```python
from build123d import *

# Parameters (mm, degrees)
F1_DEPTH = 10
F2_R     = 4
F3_R     = 2
F4_DEPTH = 13


with BuildPart() as f1:
    # F0 (on Top) → F1 (new body)
    with BuildSketch(Plane.XY):
        with BuildLine():
            Line((44.1, 0), (71.5, 0))
            ThreePointArc((71.5, 0), (0, 30), (-71.5, 0))
            Line((-71.5, 0), (-44.1, 0))
            Line((-44.1, 0), (-44.1, 8.484979))
            ThreePointArc((-44.1, 8.484979), (0, 20), (44.1, 8.484979))
            Line((44.1, 8.484979), (44.1, 0))
        make_face()
    extrude(amount=F1_DEPTH)

    # F2
    f2_edges = [f1.edges().sort_by_distance(p)[0] for p in [
        (0, 20, 10),
        (0, 30, 10),
        (0, 20, 0),
        (0, 30, 0),
        (-44.1, 4.24249, 0),
        (-44.1, 4.24249, 10),
        (44.1, 4.24249, 0),
        (44.1, 4.24249, 10),
    ]]
    fillet(f2_edges, radius=F2_R)

    # F3 (on face) → F4 (cut)
    with BuildSketch(Plane.XZ):
        with Locations((48, 5)):
            Circle(F3_R)
        with Locations((-48, 5)):
            Circle(F3_R)
    extrude(amount=-F4_DEPTH, mode=Mode.SUBTRACT)


solid = f1.part
```
Verification items for the finished model (mm, model axes). A direction names the side the tool comes from. Coordinates: 2 decimals unless noted, no trailing zeros. Order: outer loops, then holes, each group sorted by start corner. A loop starts at its lowest first (then second) coordinate and runs counter-clockwise, first axis right, second up. Notation, with made-up numbers: (-32.5, 27) - (21.5, 27) arc R29 ccw to (21.5, 51) - close; hole circle Ø5 at (40, 56.5). An arc over 180 degrees is marked (long way). Return JSON: item names as keys, results as strings.
(1) Section check A-A, the plane y = 6. Give the number of separate pieces and of enclosed holes in the cut face, and give its area (3 significant figures).
Filled sheet:
{"separate pieces": "2", "enclosed holes": "2", "area": "359 mm^2"}
(2) Thickness scan on line 1 along Z through (x, y) = (-48, 6); line 2 along X through (y, z) = (8, 6.75); line 3 along X through (y, z) = (3, 9). Record the ranges inside material, lowest first.
Filled sheet:
{"line 1": "z = 0 to 3, 7 to 10", "line 2": "x = -62.54 to -48.97, -47.03 to -44.17, 44.17 to 47.03, 48.97 to 62.54", "line 3": "x = -66.43 to -45.45, 45.45 to 66.43"}
(3) Mould release check, pull along X, two halves, no side actions. Record for faces 4 (the flat face through (-48, 13, 5)), 5 (the cylindrical face through (1.115, 29.994, 4.986)), 6 (the flat face through (0, 25, 10)), 7 (the cylindrical face through (-0.6, 20, 5)): pulls with the +X half, pulls with the -X half, needs draft (parallel to the pull), parting line crosses it, or undercut.
Filled sheet:
{"face 4": "undercut", "face 5": "parting line crosses it", "face 6": "needs draft", "face 7": "undercut"}
(4) Go/stop test with flat-tipped pins: pin 1 (2.5 mm diameter, centred on x = 48, z = 5, fed in from -Y); pin 2 (2.5 mm diameter, centred on x = -48, z = 5, fed in from +Y); pin 3 (3 mm diameter, centred on x = -17.5, z = 6.5, fed in from +Y). Record where each tip stops, or that it passes through.
Filled sheet:
{"pin 1": "stops at y = 13", "pin 2": "stops at y = 18.43", "pin 3": "stops at y = 28.7"}
(5) Section check B-B, the plane z = 1.25. Record the cut outline in (x, y).
Filled sheet:
{"outline": "(-69.96, 0) - (-45.2, 0) - (-45.2, 9.12) arc R91.3 cw to (45.2, 9.12) - (45.2, 0) - (69.96, 0) arc R99.11 ccw to start"}
(6) Access from +Z, -Z, +X, -X, +Y, -Y to the whole of each face (thin tool, end or side, straight path). Record for faces 1 (the cylindrical face through (-45.241, 4.273, 1.203)), 2 (the cylindrical face through (45.241, 4.122, 8.797)), 3 (the cylindrical face through (-50, 6, 5)).
Filled sheet:
{"face 1": "-Z, -Y", "face 2": "+Z, -Y", "face 3": "-Y"}
